Can you work these out from the model? Positions are in its coordinate system, mm. Face numbers are marked on the shaded views. A direction names the side the tool comes from. Round coordinates to 2 decimals unless told otherwise and drop trailing zeros. Loops run counter-clockwise (first coordinate to the right, second up) from the corner with the lowest first, then second, coordinate; pieces in that order, holes last. Notation, with made-up numbers: (81, 75.25) -> (87, 75.25) arc R25 cw to (87, 101.25) -> close; hole circle Ø9 at (-38.5, 65.5). An arc over 180 degrees is marked (long way). Use a Markdown table: item, result.
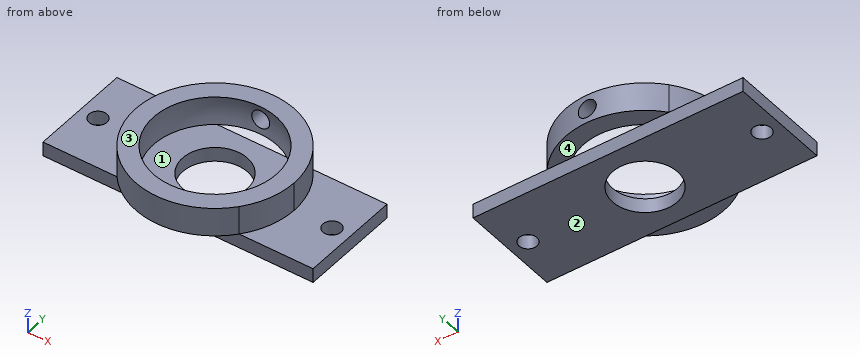
from build123d import *

# Parameters (mm, degrees)
F0_W     = 95.25
F0_H     = 35.56
F0_R     = 3.175
F0_R_2   = 11.43
F1_DEPTH = 5.08
F2_R     = 11.43
F3_DEPTH = 10.16
F8_D     = 6.35
F8_DEPTH = 27.941


with BuildPart() as f1:
    # F0 (on Top) → F1 (new body)
    with BuildSketch(Plane.XY):
        with Locations((-41.275, 0)):
            Rectangle(F0_W, F0_H)
        with Locations((-82.55, 0)):
            Circle(F0_R, mode=Mode.SUBTRACT)
        with Locations((-41.275, 0)):
            Circle(F0_R_2, mode=Mode.SUBTRACT)
        Circle(F0_R, mode=Mode.SUBTRACT)
    extrude(amount=F1_DEPTH)

    # F2 (on face) → F3 (join)
    with BuildSketch(Plane.XY.offset(5.08)):
        with BuildLine():
            ThreePointArc((-19.7223853094, -17.78), (-14.9802889876, -9.4462570774), (-13.335, 0))
            ThreePointArc((-13.335, 0), (-14.9802889876, 9.4462570774), (-19.7223853094, 17.78))
            Line((-19.7223853094, 17.78), (-62.8276146906, 17.78))
            ThreePointArc((-62.8276146906, 17.78), (-69.215, 0), (-62.8276146906, -17.78))
            Line((-62.8276146906, -17.78), (-19.7223853094, -17.78))
        make_face()
        with Locations((-41.275, 0)):
            Circle(F2_R, mode=Mode.SUBTRACT)
        with BuildLine():
            Line((-62.8276146906, 17.78), (-19.7223853094, 17.78))
            ThreePointArc((-19.7223853094, 17.78), (-41.275, 27.94), (-62.8276146906, 17.78))
        make_face()
        with BuildLine():
            ThreePointArc((-62.8276146906, -17.78), (-41.275, -27.94), (-19.7223853094, -17.78))
            Line((-19.7223853094, -17.78), (-62.8276146906, -17.78))
        make_face()
    extrude(amount=F3_DEPTH)

    # F5 (on offset) → F6 (revolve, cut)
    with BuildSketch(Plane.YZ.offset(-41.275)):
        Polygon((0, 5.08), (0, 10.16), (-21.6366407975, 5.08), align=None)
        with BuildLine():
            Line((-21.6366407975, 5.08), (0, 10.16))
            Line((0, 10.16), (0, 32.385))
            ThreePointArc((0, 32.385), (-17.4191507399, 23.9630363507), (-21.6366407975, 5.08))
        make_face()
    revolve(axis=Axis((-41.275, 0, 21.2725), (0, 0, 1)), mode=Mode.SUBTRACT)

    # F8 (through all, one way)
    with BuildSketch(Plane.XZ):
        with Locations((-41.275, 10.16)):
            Circle(F8_D / 2)
    extrude(amount=-F8_DEPTH, mode=Mode.SUBTRACT)


solid = f1.part
1. Will these pins go through, and if not, where does the flat tip stop? pin 1 Ø4 at (y, z) = (-9.5, 12) entering from -X; pin 2 Ø4 at (y, z) = (3, 10.5) entering from +X; pin 3 Ø8 at (x, z) = (-78.5, 11.5) entering from +Y; pin 4 Ø4 at (x, z) = (-41, 3) entering from +Y.
Answer sheet:
| item | result |
|---|---|
| pin 1 | stops at x = -68.19 |
| pin 2 | stops at x = -13.35 |
| pin 3 | passes through |
| pin 4 | stops at y = 17.78 |
2. Which directions (+Z, -Z, +X, -X, +Y, -Y) give clear straight access to the entire face, cutting with the end or side of a thin tool? Please do the marked faces 3 and 4.
Answer sheet:
| item | result |
|---|---|
| face 3 | +Z, +X, -X, +Y, -Y |
| face 4 | -Z, +X, -X, +Y |
3. I want a section at C-C (x = -34.5). Please give me the cut outline in (y, z).
Answer sheet:
| item | result |
|---|---|
| outline | (-27.11, 5.08) -> (-20.55, 5.08) arc R21.17 cw to (-20.55, 15.24) -> (-27.11, 15.24) -> close; (-17.78, 0) -> (-9.21, 0) -> (-9.21, 5.08) -> (-17.78, 5.08) -> close; (9.21, 0) -> (17.78, 0) -> (17.78, 5.08) -> (9.21, 5.08) -> close; (20.55, 5.08) -> (27.11, 5.08) -> (27.11, 15.24) -> (20.55, 15.24) arc R21.17 cw to start |
4. I want a section at A-A (x = -82.55). Please give me the cut outline in (y, z) (3 decimals).
Answer sheet:
| item | result |
|---|---|
| outline | (-17.78, 0) -> (-3.175, 0) -> (-3.175, 5.08) -> (-17.78, 5.08) -> close; (3.175, 0) -> (17.78, 0) -> (17.78, 5.08) -> (3.175, 5.08) -> close |
5. If we mould it in two halves opening along Y, with no side actions, what happens to the marked faces 1 and 2? For each: +Y half, -Y half, draft (parallel to the pull), parting line (faces both ways), or undercut.
Answer sheet:
| item | result |
|---|---|
| face 1 | undercut |
| face 2 | draft |
6. I need wall thicknesses on line 1 (Y direction, x = -82.55, z = 2.75) (3 decimals); line 2 (Z direction, x = -58, y = -20); line 3 (X direction, y = 13.5, z = 10.5). Which ranges of each line are inside material? Lowest first, please.
Answer sheet:
| item | result |
|---|---|
| line 1 | y = -17.78 to -3.175, 3.175 to 17.78 |
| line 2 | z = 5.08 to 15.24 |
| line 3 | x = -65.74 to -58.93, -23.62 to -16.81 |
7. I want a section at D-D (y = -1). State how many separate pieces and enclosed holes the cut face has, plus the area to 3 significant figures.
Answer sheet:
| item | result |
|---|---|
| separate pieces | 4 |
| enclosed holes | 0 |
| area | 427 mm² |
8. I want a section at B-B (z = 1). Please give me the cut outline in (x, y) (3 decimals), plus the area to 3 significant figures.
Answer sheet:
| item | result |
|---|---|
| outline | (-88.9, -17.78) -> (6.35, -17.78) -> (6.35, 17.78) -> (-88.9, 17.78) -> close; hole circle Ø6.35 at (-82.55, 0); hole circle Ø22.86 at (-41.275, 0); hole circle Ø6.35 at (0, 0) |
| area | 2,910 mm² |
